Verification items for the finished model (mm, model axes). A direction names the side the tool comes from. Give positions to 0.01 mm unless a question says otherwise; leave off trailing zeros. Write each loop counter-clockwise with the first axis right and the second up, starting at its lowest first coordinate (ties: lowest second). Pieces come first, ordered by that corner, then holes. Notation, with made-up numbers: (44.5, 41) - (78.5, 41) arc R21 ccw to (78.5, 57) - close; hole circle Ø7 at (80, 83). An arc over 180 degrees is marked (long way). Put each result on its own line as item: value.
from build123d import *

# Parameters (mm, degrees)
RESSALTO_EXTRUS_O1_DEPTH = 28
ESBO_O2_W                = 280
ESBO_O2_H                = 52
CORTE_EXTRUS_O1_DEPTH    = 23
FILETE6_R                = 5
RESSALTO_EXTRUS_O2_DEPTH = 10
ESBO_O4_R                = 2
CORTE_EXTRUS_O3_DEPTH    = 357.192363759
ESBO_O5_R                = 2
CORTE_EXTRUS_O4_DEPTH    = 357.192363759
ESBO_O6_R                = 2.25
CORTE_EXTRUS_O5_DEPTH    = 356.76537212
ESBO_O7_R                = 2.5
CORTE_EXTRUS_O6_DEPTH    = 10
ESBO_O13_R               = 2
CORTE_EXTRUS_O12_DEPTH   = 357.192363759
ESBO_O15_W               = 30
ESBO_O15_H               = 10
CORTE_EXTRUS_O13_DEPTH   = 4
ESBO_O16_R               = 0.75
CORTE_EXTRUS_O14_DEPTH   = 318.376747731
FILETE7_R                = 5
ESBO_O17_R               = 2
CORTE_EXTRUS_O15_DEPTH   = 10


with BuildPart() as part:
    # Esboço1 → Ressalto-extrusão1 (new body)
    with BuildSketch(Plane.XY):
        Polygon((350, 30), (290, 30), (290, 62), (0, 62), (0, 0), (290, 0), (350, 0), align=None)
    extrude(amount=RESSALTO_EXTRUS_O1_DEPTH)

    # Esboço2 → Corte-extrusão1 (cut)
    with BuildSketch(Plane(origin=(0, 0, 0), x_dir=(-1, 0, 0), z_dir=(0, 0, -1))):
        with Locations((-145, 31)):
            Rectangle(ESBO_O2_W, ESBO_O2_H)
    extrude(amount=-CORTE_EXTRUS_O1_DEPTH, mode=Mode.SUBTRACT)

    # Filete6
    filete6_edges = [part.edges().sort_by_distance(p)[0] for p in [
        (285, 5, 11.5),
        (285, 57, 11.5),
        (5, 57, 11.5),
        (5, 5, 11.5),
    ]]
    fillet(filete6_edges, radius=FILETE6_R)

    # Esboço3 → Ressalto-extrusão2 (add)
    with BuildSketch(Plane(origin=(0, 0, 23), x_dir=(-1, 0, 0), z_dir=(0, 0, -1))):
        with BuildLine():
            Line((-272, 30), (-272, 57))
            Line((-272, 57), (-280, 57))
            ThreePointArc((-280, 57), (-283.535533906, 55.535533906), (-285, 52))
            Line((-285, 52), (-285, 10))
            ThreePointArc((-285, 10), (-283.535533906, 6.464466094), (-280, 5))
            Line((-280, 5), (-272, 5))
            Line((-272, 5), (-272, 30))
        make_face()
    extrude(amount=RESSALTO_EXTRUS_O2_DEPTH)

    # Esboço4 → Corte-extrusão3 (cut, through all)
    with BuildSketch(Plane(origin=(0, 0, 23), x_dir=(-1, 0, 0), z_dir=(0, 0, -1))):
        with Locations((-72.2, 10)):
            Circle(ESBO_O4_R)
        with Locations((-72.2, 52)):
            Circle(ESBO_O4_R)
    extrude(amount=-CORTE_EXTRUS_O3_DEPTH, mode=Mode.SUBTRACT)

    # Esboço5 → Corte-extrusão4 (cut, through all)
    with BuildSketch(Plane(origin=(0, 0, 23), x_dir=(-1, 0, 0), z_dir=(0, 0, -1))):
        with Locations((-264.5, 52)):
            Circle(ESBO_O5_R)
        with Locations((-264.5, 10)):
            Circle(ESBO_O5_R)
    extrude(amount=-CORTE_EXTRUS_O4_DEPTH, mode=Mode.SUBTRACT)

    # Esboço6 → Corte-extrusão5 (cut, through all)
    with BuildSketch(Plane(origin=(0, 0, 13), x_dir=(-1, 0, 0), z_dir=(0, 0, -1))):
        with Locations((-278.5, 10)):
            Circle(ESBO_O6_R)
        with Locations((-278.5, 52)):
            Circle(ESBO_O6_R)
    extrude(amount=-CORTE_EXTRUS_O5_DEPTH, mode=Mode.SUBTRACT)

    # Esboço7 → Corte-extrusão6 (cut)
    with BuildSketch(Plane(origin=(0, 0, 23), x_dir=(-1, 0, 0), z_dir=(0, 0, -1))):
        with Locations((-60, 48.7)):
            Circle(ESBO_O7_R)
        with Locations((-60, 13.3)):
            Circle(ESBO_O7_R)
    extrude(amount=-CORTE_EXTRUS_O6_DEPTH, mode=Mode.SUBTRACT)

    # Esboço13 → Corte-extrusão12 (cut, through all)
    with BuildSketch(Plane(origin=(0, 0, 23), x_dir=(-1, 0, 0), z_dir=(0, 0, -1))):
        with Locations((-29, 46.5)):
            Circle(ESBO_O13_R)
        with Locations((-29, 31)):
            Circle(ESBO_O13_R)
        with Locations((-29, 15.5)):
            Circle(ESBO_O13_R)
    extrude(amount=-CORTE_EXTRUS_O12_DEPTH, mode=Mode.SUBTRACT)

    # Esboço15 → Corte-extrusão13 (cut)
    with BuildSketch(Plane(origin=(0, 0, 0), x_dir=(-1, 0, 0), z_dir=(0, 0, -1))):
        with Locations((-295, 13)):
            Rectangle(ESBO_O15_W, ESBO_O15_H)
    extrude(amount=-CORTE_EXTRUS_O13_DEPTH, mode=Mode.SUBTRACT)

    # Esboço16 → Corte-extrusão14 (cut, through all)
    with BuildSketch(Plane.ZY.offset(-310)):
        with Locations((0, 13)):
            Circle(ESBO_O16_R)
    extrude(amount=-CORTE_EXTRUS_O14_DEPTH, mode=Mode.SUBTRACT)

    # Filete7
    # the kernel refuses this fillet: 5 mm, written as the material it adds along each edge
    with BuildSketch(Plane(origin=(310, 18, 0), x_dir=(-1, 0, 0), z_dir=(0, 0, 1))) as filete7_piece_1_section:
        with BuildLine():
            CenterArc((FILETE7_R, FILETE7_R), FILETE7_R, 180, 90)
            Line((0, FILETE7_R), (0, 0))
            Line((0, 0), (FILETE7_R, 0))
        make_face()
    filete7_piece_1 = extrude(amount=16.5, mode=Mode.PRIVATE)
    filete7_piece_1 = filete7_piece_1 - Plane(origin=(308.865698772, 13, 0), x_dir=(0, 0, 1), z_dir=(-1, 0, 0)) * Cylinder(0.75, 53, mode=Mode.PRIVATE)
    add(filete7_piece_1)
    with BuildSketch(Plane(origin=(310, 8, 0), x_dir=(-1, 0, 0), z_dir=(0, 0, 1))) as filete7_piece_2_section:
        with BuildLine():
            CenterArc((FILETE7_R, -FILETE7_R), FILETE7_R, 90, 90)
            Line((0, -FILETE7_R), (0, 0))
            Line((0, 0), (FILETE7_R, 0))
        make_face()
    filete7_piece_2 = extrude(amount=16.5, mode=Mode.PRIVATE)
    filete7_piece_2 = filete7_piece_2 - Plane(origin=(308.865698858, 13, 0), x_dir=(0, 0, 1), z_dir=(-1, 0, 0)) * Cylinder(0.75, 54, mode=Mode.PRIVATE)
    add(filete7_piece_2)

    # Esboço17 → Corte-extrusão15 (cut)
    with BuildSketch(Plane(origin=(0, 0, 0), x_dir=(-1, 0, 0), z_dir=(0, 0, -1))):
        with Locations((-294.791287847, 4)):
            Circle(ESBO_O17_R)
        with Locations((-295, 22)):
            Circle(ESBO_O17_R)
    extrude(amount=-CORTE_EXTRUS_O15_DEPTH, mode=Mode.SUBTRACT)


solid = part.part
Q1. Section check A-A, the plane x = 101.5. Record the cut outline in (y, z), plus the area to 3 significant figures.
Answers follow:
outline: (0, 0) - (5, 0) - (5, 23) - (57, 23) - (57, 0) - (62, 0) - (62, 28) - (0, 28) - close
area: 540 mm2
Q2. Go/stop test with flat-tipped pins: pin 1 Ø12 at (x, y) = (235, 25.5) entering from -Z; pin 2 Ø14 at (y, z) = (42, 16) entering from +X; pin 3 Ø3 at (x, y) = (294.79, 4) entering from -Z. Record where each tip stops, or that it passes through.
Answers follow:
pin 1: stops at z = 23
pin 2: stops at x = 290
pin 3: stops at z = 10
Q3. Release check for a two-part mould opening along X. For faces 1 (the face through (279, 31, 13)), 2 (the face through (290, 46, 14)), 3 (the face through (147, 62, 14)), 4 (the face through (0, 31, 14)) record: released by +X, released by -X, zero draft, split by the parting line, or undercut.
Answers follow:
face 1: undercut
face 2: released by +X
face 3: zero draft
face 4: released by -X
Q4. Set-up check for faces 5 (the face through (173, 0, 14)), 6 (the face through (320, 30, 14)), 7 (the face through (285, 31, 6)): record each of +Z, -Z, +X, -X, +Y, -Y from which the full face is reachable in a straight line by a thin tool's end or side.
Answers follow:
face 5: +Z, -Z, +X, -X, -Y
face 6: +Z, -Z, +X, +Y
face 7: -Z
Q5. Scan lines: line 1 along Y through (x, z) = (278.5, 21.75); line 2 along Y through (x, z) = (72.2, 27.05); line 3 along X through (y, z) = (7, 19). Record each from-to range of solid material in increasing order.
Answers follow:
line 1: y = 0 to 7.75, 12.25 to 49.75, 54.25 to 62
line 2: y = 0 to 8, 12 to 50, 54 to 62
line 3: x = 0 to 6, 272 to 350
